```python
from build123d import *

# Parameters (mm, degrees)
F0_R     = 11.325
F1_DEPTH = 11


with BuildPart() as f1:
    # F0 (on Top) → F1 (new body)
    with BuildSketch(Plane.XY):
        with BuildLine():
            ThreePointArc((11.016607, -6.901766), (12.494316, -3.590551), (13, 0))
            ThreePointArc((13, 0), (12.494316, 3.590551), (11.016607, 6.901766))
            ThreePointArc((11.016607, 6.901766), (6.5, 11.25833), (0.468801, 12.991544))
            ThreePointArc((0.468801, 12.991544), (-6.5, 11.25833), (-11.485408, 6.089778))
            ThreePointArc((-11.485408, 6.089778), (-13, 0), (-11.485408, -6.089778))
            ThreePointArc((-11.485408, -6.089778), (-6.5, -11.25833), (0.468801, -12.991544))
            ThreePointArc((0.468801, -12.991544), (6.5, -11.25833), (11.016607, -6.901766))
        make_face()
        Circle(F0_R, mode=Mode.SUBTRACT)
        with BuildLine():
            ThreePointArc((0.468801, 12.991544), (6.5, 11.25833), (11.016607, 6.901766))
            ThreePointArc((11.016607, 6.901766), (18.941923, 8.670001), (24.784471, 14.309321))
            ThreePointArc((24.784471, 14.309321), (17.226452, 17.164186), (14.24508, 24.673203))
            ThreePointArc((14.24508, 24.673203), (6.251395, 23.500638), (0, 28.618642))
            ThreePointArc((0, 28.618642), (-1.962521, 20.739187), (0.468801, 12.991544))
        make_face()
        with BuildLine():
            ThreePointArc((24.784471, -14.309321), (18.941923, -8.670001), (11.016607, -6.901766))
            ThreePointArc((11.016607, -6.901766), (6.5, -11.25833), (0.468801, -12.991544))
            ThreePointArc((0.468801, -12.991544), (-1.962521, -20.739187), (0, -28.618642))
            ThreePointArc((0, -28.618642), (6.251395, -23.500638), (14.24508, -24.673203))
            ThreePointArc((14.24508, -24.673203), (17.226452, -17.164186), (24.784471, -14.309321))
        make_face()
        with BuildLine():
            ThreePointArc((-11.485408, -6.089778), (-13, 0), (-11.485408, 6.089778))
            ThreePointArc((-11.485408, 6.089778), (-16.979402, 12.069187), (-24.784471, 14.309321))
            ThreePointArc((-24.784471, 14.309321), (-23.477847, 6.336452), (-28.490161, 0))
            ThreePointArc((-28.490161, 0), (-23.477847, -6.336452), (-24.784471, -14.309321))
            ThreePointArc((-24.784471, -14.309321), (-16.979402, -12.069187), (-11.485408, -6.089778))
        make_face()
    extrude(amount=F1_DEPTH)


solid = f1.part
```
Source: CAD feature listing. Evaluate the final solid. Frame: model axes, mm. Coordinates: 2 decimals unless noted, no trailing zeros. Loops run counter-clockwise (first coordinate to the right, second up) from the corner with the lowest first, then second, coordinate; pieces in that order, holes last. Notation, with made-up numbers: (81.25, 24) -> (127.25, 24) arc R25 ccw to (127.25, 60) -> close; hole circle Ø5 at (2, -38.5). An arc over 180 degrees is marked (long way). One line per item, written item: value. Start each with the question number.
Q1. Section query C-C, the plane y = -4.5. Return the cut outline in (x, z).
Q2. Section query D-D, the plane y = 19. Return the cut outline in (x, z).
Q3. Contact query for flat-ended pins moving along their axis: P1, Ø1, axis at x = 5, y = -8, coming from the -Z side; P2, Ø5, axis at x = -18.5, y = -14.5, coming from the +Z side; P3, Ø2, axis at y = 20, z = 3.5, coming from the +X side; P4, Ø2, axis at y = -9, z = 8, coming from the -X side. Output: stop coordinate, or through.
Q4. Section query B-B, the plane x = -4.5. Return the cut outline in (y, z), and give its area (3 significant figures).
Q5. Mould query, pull axis Y, two halves, no side actions, for faces 1 (the face through (6.139, -23.532, 5.423)), 2 (the face through (-2.455, -11.056, 5.423)), 3 (the face through (-6, -10, 0)). Classes: pulls with the +Y half, pulls with the -Y half, needs draft (parallel to the pull), parting line crosses it, or undercut.
Q6. Line query: line 1 along X through (y, z) = (-5.5, 8.5); line 2 along Y through (x, z) = (17, 8.5); line 3 along X through (y, z) = (-3.5, 3.25). Output: solid intervals per line, ascending.
Results:
1. outline: (-24.15, 0) -> (-10.39, 0) -> (-10.39, 11) -> (-24.15, 11) -> close; (10.39, 0) -> (12.2, 0) -> (12.2, 11) -> (10.39, 11) -> close
2. outline: (-1.81, 0) -> (15.75, 0) -> (15.75, 11) -> (-1.81, 11) -> close
3. P1: through
3. P2: z = 11
3. P3: x = 15.75
3. P4: x = -23.23
4. outline: (-12.2, 0) -> (-10.39, 0) -> (-10.39, 11) -> (-12.2, 11) -> close; (10.39, 0) -> (12.2, 0) -> (12.2, 11) -> (10.39, 11) -> close
4. area: 39.7 mm^2
5. face 1: pulls with the -Y half
5. face 2: undercut
5. face 3: needs draft
6. line 1: -23.73 to -9.9, 9.9 to 11.78
6. line 2: -17.39 to -7.8, 7.8 to 17.39
6. line 3: -24.71 to -10.77, 10.77 to 12.52
